```python
from build123d import *

# Parameters (mm, degrees)
SKETCH1_R           = 2
SKETCH1_R_2         = 2.5
SKETCH1_W           = 33
SKETCH1_H           = 80
SKETCH1_W_2         = 26.358753283
SKETCH1_H_2         = 29.759882739
BOSS_EXTRUDE1_DEPTH = 5


with BuildPart() as part:
    # Sketch1 → Boss-Extrude1 (new body)
    with BuildSketch(Plane.XY):
        with BuildLine():
            Line((-125.940029712, -95.672909388), (-104.635809021, -95.672909388))
            ThreePointArc((-104.635809021, -95.672909388), (-100.405628635, -98.00728115), (-96.175448249, -95.672909388))
            Line((-96.175448249, -95.672909388), (-69.744751877, -95.672909388))
            ThreePointArc((-69.744751877, -95.672909388), (-65.514571491, -98.00728115), (-61.284391105, -95.672909388))
            Line((-61.284391105, -95.672909388), (-39.980170414, -95.672909388))
            Line((-39.980170414, -95.672909388), (-23.23481866, -66.66910936))
            ThreePointArc((-23.23481866, -66.66910936), (-20.75474442, -64.873494769), (-20.439733688, -61.827880177))
            Line((-20.439733688, -61.827880177), (-5.339154263, -35.672909388))
            Line((-5.339154263, -35.672909388), (68.561680194, -35.672909388))
            Line((68.561680194, -35.672909388), (83.651079822, -61.808516201))
            ThreePointArc((83.651079822, -61.808516201), (83.885152959, -65.076529173), (86.598298645, -66.913248943))
            Line((86.598298645, -66.913248943), (103.202696345, -95.672909388))
            Line((103.202696345, -95.672909388), (124.216145364, -95.672909388))
            ThreePointArc((124.216145364, -95.672909388), (128.736262965, -98.535495794), (133.256380567, -95.672909388))
            Line((133.256380567, -95.672909388), (159.108871421, -95.672909388))
            ThreePointArc((159.108871421, -95.672909388), (163.628989022, -98.535495794), (168.149106623, -95.672909388))
            Line((168.149106623, -95.672909388), (189.162555642, -95.672909388))
            Line((189.162555642, -95.672909388), (189.162555642, 95.180535099))
            Line((189.162555642, 95.180535099), (113.042402195, 95.180535099))
            ThreePointArc((113.042402195, 95.180535099), (108.712275177, 97.680535099), (104.382148158, 95.180535099))
            Line((104.382148158, 95.180535099), (-41.159528738, 95.180535099))
            ThreePointArc((-41.159528738, 95.180535099), (-45.489655757, 97.680535099), (-49.819782776, 95.180535099))
            Line((-49.819782776, 95.180535099), (-125.940029712, 95.180535099))
            Line((-125.940029712, 95.180535099), (-125.940029712, -95.672909388))
        make_face()
        with Locations((67.611262965, 29.327090612)):
            Circle(SKETCH1_R, mode=Mode.SUBTRACT)
        with Locations((36.611262965, 29.327090612)):
            Circle(SKETCH1_R, mode=Mode.SUBTRACT)
        with Locations((26.611262965, 29.327090612)):
            Circle(SKETCH1_R, mode=Mode.SUBTRACT)
        with Locations((-4.388737035, 29.327090612)):
            Circle(SKETCH1_R, mode=Mode.SUBTRACT)
        with Locations((67.611262965, -5.672909388)):
            Circle(SKETCH1_R, mode=Mode.SUBTRACT)
        with Locations((36.611262965, -5.672909388)):
            Circle(SKETCH1_R, mode=Mode.SUBTRACT)
        with Locations((26.611262965, -5.672909388)):
            Circle(SKETCH1_R, mode=Mode.SUBTRACT)
        with Locations((-4.388737035, -5.672909388)):
            Circle(SKETCH1_R, mode=Mode.SUBTRACT)
        with Locations((-61.588737035, -13.672909388)):
            Circle(SKETCH1_R_2, mode=Mode.SUBTRACT)
        with Locations((-61.588737035, 37.327090612)):
            Circle(SKETCH1_R_2, mode=Mode.SUBTRACT)
        with Locations((124.811262965, 37.327090612)):
            Circle(SKETCH1_R_2, mode=Mode.SUBTRACT)
        with Locations((124.811262965, -13.672909388)):
            Circle(SKETCH1_R_2, mode=Mode.SUBTRACT)
        with Locations((-24.888737035, 11.827090612)):
            Rectangle(SKETCH1_W, SKETCH1_H, mode=Mode.SUBTRACT)
        with Locations((88.111262965, 11.827090612)):
            Rectangle(SKETCH1_W, SKETCH1_H, mode=Mode.SUBTRACT)
        with BuildLine():
            Line((144.581262965, -34.665729578), (147.181262965, -34.665729578))
            ThreePointArc((147.181262965, -34.665729578), (150.716796871, -33.201263484), (152.181262965, -29.665729578))
            Line((152.181262965, -29.665729578), (152.181262965, 53.319910802))
            ThreePointArc((152.181262965, 53.319910802), (150.716796871, 56.855444707), (147.181262965, 58.319910802))
            Line((147.181262965, 58.319910802), (144.581262965, 58.319910802))
            ThreePointArc((144.581262965, 58.319910802), (141.04572906, 56.855444707), (139.581262965, 53.319910802))
            Line((139.581262965, 53.319910802), (139.581262965, -29.665729578))
            ThreePointArc((139.581262965, -29.665729578), (141.04572906, -33.201263484), (144.581262965, -34.665729578))
        make_face(mode=Mode.SUBTRACT)
        with BuildLine():
            Line((-83.958737035, -34.665729578), (-81.358737035, -34.665729578))
            ThreePointArc((-81.358737035, -34.665729578), (-77.823203129, -33.201263484), (-76.358737035, -29.665729578))
            Line((-76.358737035, -29.665729578), (-76.358737035, 53.319910802))
            ThreePointArc((-76.358737035, 53.319910802), (-77.823203129, 56.855444707), (-81.358737035, 58.319910802))
            Line((-81.358737035, 58.319910802), (-83.958737035, 58.319910802))
            ThreePointArc((-83.958737035, 58.319910802), (-87.49427094, 56.855444707), (-88.958737035, 53.319910802))
            Line((-88.958737035, 53.319910802), (-88.958737035, -29.665729578))
            ThreePointArc((-88.958737035, -29.665729578), (-87.49427094, -33.201263484), (-83.958737035, -34.665729578))
        make_face(mode=Mode.SUBTRACT)
        with Locations((52.23838386, 11.97050865)):
            Rectangle(SKETCH1_W_2, SKETCH1_H_2, mode=Mode.SUBTRACT)
        with Locations((10.98423556, 11.97050865)):
            Rectangle(SKETCH1_W_2, SKETCH1_H_2, mode=Mode.SUBTRACT)
    extrude(amount=BOSS_EXTRUDE1_DEPTH)


solid = part.part
```
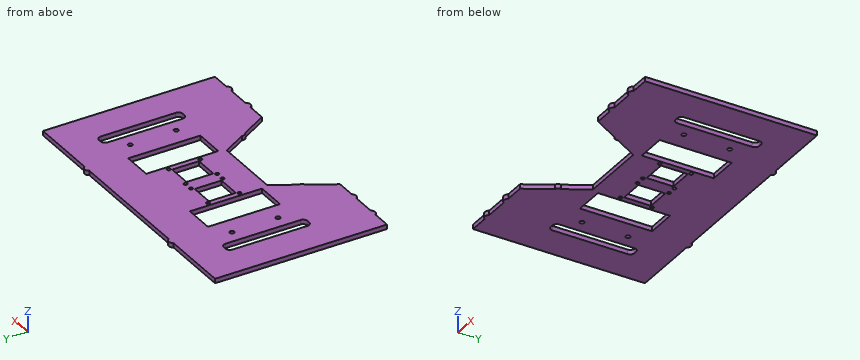
Geometry: final body of the model. Coordinates: model frame, mm. Round coordinates to 2 decimals unless told otherwise and drop trailing zeros. Write each loop counter-clockwise with the first axis right and the second up, starting at its lowest first coordinate (ties: lowest second). Pieces come first, ordered by that corner, then holes. Notation, with made-up numbers: M 13,-29.75 L 42,-29.75 A8 cw 42,-17.75 Z; hole C -29.75,-8 d11. An arc over 180 degrees is marked long. Answer in a Markdown table with one row per item. Add a question column.
(1) Cut plane D-D, the plane z = 2.8. Give the number of separate pieces and of enclosed holes in the cut face, then the cut area to 3 significant figures.
(2) Cut plane A-A, the plane y = 3. Return the cut outline in (x, z).
(3) Contact query for flat-ended pins moving along their axis: pin 1 (1.5 mm diameter, centred on x = 83, z = 2.5, fed in from +Y); pin 2 (1.5 mm diameter, centred on x = 92.5, y = 64, fed in from -Z); pin 3 (2.5 mm diameter, centred on x = -28.5, z = 1.5, fed in from -Y). Output: stop coordinate, or through.
(4) Ray query, L1, parallel to X at y = -28.5, z = 3.2; L2, parallel to Y at x = -84, z = 1.7; L3, parallel to Y at x = -63.5, z = 0.9. Return the intervals inside material, ascending.
(5) Cut plane B-B, the plane x = 17.5. Return the cut outline in (y, z), then the cut area to 3 significant figures.
(6) Cut plane C-C, the plane y = -83.5. Return the cut outline in (x, z).
Established:
| question | item | result |
|---|---|---|
| 1 | separate pieces | 1 |
| 1 | enclosed holes | 18 |
| 1 | area | 44,400 mm² |
| 2 | outline | M -125.94,0 L -88.96,0 L -88.96,5 L -125.94,5 Z; M -76.36,0 L -41.39,0 L -41.39,5 L -76.36,5 Z; M -8.39,0 L -2.2,0 L -2.2,5 L -8.39,5 Z; M 24.16,0 L 39.06,0 L 39.06,5 L 24.16,5 Z; M 65.42,0 L 71.61,0 L 71.61,5 L 65.42,5 Z; M 104.61,0 L 139.58,0 L 139.58,5 L 104.61,5 Z; M 152.18,0 L 189.16,0 L 189.16,5 L 152.18,5 Z |
| 3 | pin 1 | y = 95.18 |
| 3 | pin 2 | z = 0 |
| 3 | pin 3 | y = -77.95 |
| 4 | L1 | -125.94 to -88.96, -76.36 to 139.58, 152.18 to 189.16 |
| 4 | L2 | -95.67 to -34.67, 58.32 to 95.18 |
| 4 | L3 | -97.58 to -15.28, -12.06 to 35.72, 38.94 to 95.18 |
| 5 | outline | M -35.67,0 L -2.91,0 L -2.91,5 L -35.67,5 Z; M 26.85,0 L 95.18,0 L 95.18,5 L 26.85,5 Z |
| 5 | area | 505 mm² |
| 6 | outline | M -125.94,0 L -32.95,0 L -32.95,5 L -125.94,5 Z; M 96.17,0 L 189.16,0 L 189.16,5 L 96.17,5 Z |
